Geometry check sheet. Reference: drawing and pictorial views, mm from the part's lowest x, y, z. A direction names the side the tool comes from. Round coordinates to 2 decimals unless told otherwise and drop trailing zeros. Write each loop counter-clockwise with the first axis right and the second up, starting at its lowest first coordinate (ties: lowest second). Pieces come first, ordered by that corner, then holes. Notation, with made-up numbers: (46, 83.5) -> (62, 83.5) arc R19 ccw to (62, 95.5) -> close; hole circle Ø1 at (62.5, 82.5). An arc over 180 degrees is marked (long way). Answer as a JSON object with one key per item and string values. Group by question number.
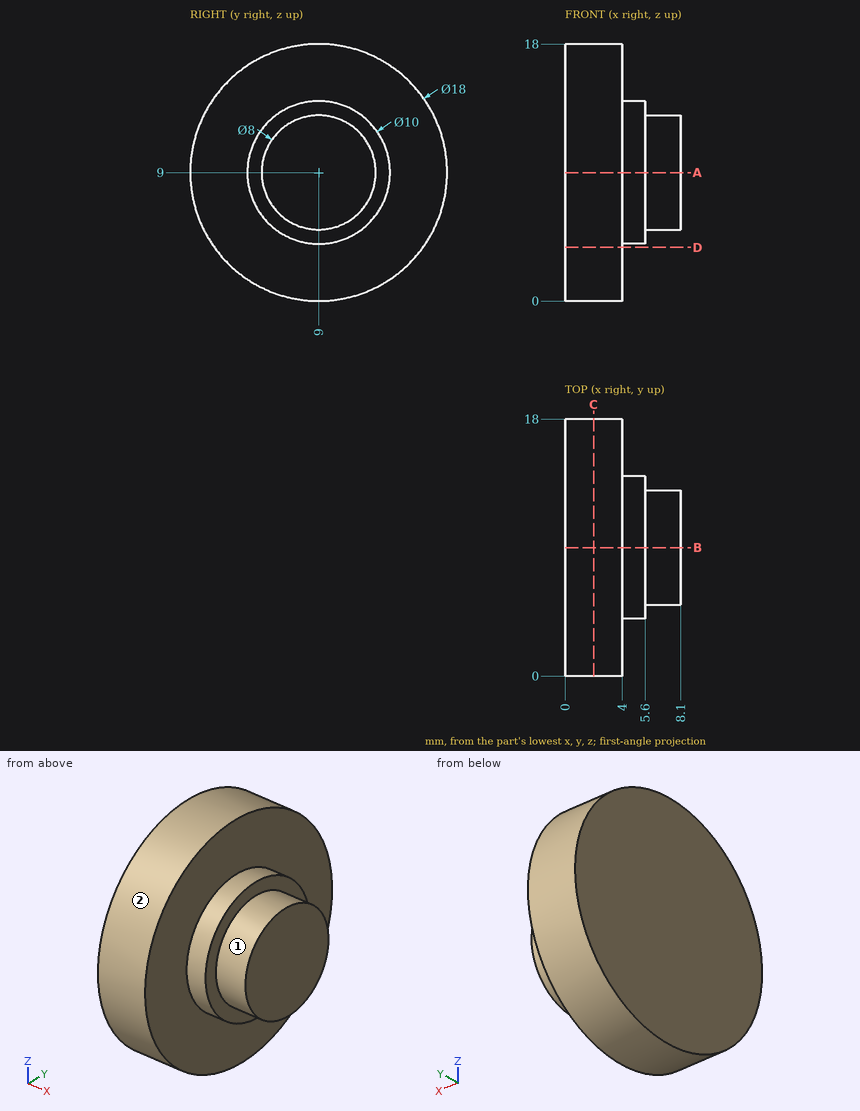
(1) Section check A-A on z = 9. Record the cut outline in (x, y).
(2) Access from +Z, -Z, +X, -X, +Y, -Y to the whole of each face (thin tool, end or side, straight path). Record for the marked faces 1 and 2.
(3) Go/stop test with flat-tipped pins: pin 1 Ø3 at (y, z) = (16, 4) entering from +X; pin 2 Ø3 at (x, y) = (6.5, 8) entering from -Z; pin 3 Ø4 at (x, y) = (4, 14.5) entering from -Z. Record where each tip stops, or that it passes through.
(4) Scan lines: line 1 along X through (y, z) = (11.25, 13.25); line 2 along X through (y, z) = (5.25, 12.5); line 3 along Z through (x, y) = (7, 12.25). Record each from-to range of solid material in increasing order.
(5) Section check D-D on z = 3.75. Record the cut outline in (x, y).
(6) Section check C-C on x = 2. Record the cut outline in (y, z).
Data:
{
 "1": {"outline": "(0, 0) -> (4, 0) -> (4, 4) -> (5.6, 4) -> (5.6, 5) -> (8.1, 5) -> (8.1, 13) -> (5.6, 13) -> (5.6, 14) -> (4, 14) -> (4, 18) -> (0, 18) -> close"},
 "2": {"face 1": "+X", "face 2": "+X, -X"},
 "3": {"pin 1": "stops at x = 4", "pin 2": "stops at z = 4", "pin 3": "stops at z = 0.71"},
 "4": {"line 1": "x = 0 to 5.6", "line 2": "x = 0 to 4", "line 3": "z = 6.67 to 11.33"},
 "5": {"outline": "(0, 1.69) -> (4, 1.69) -> (4, 16.31) -> (0, 16.31) -> close"},
 "6": {"outline": "circle Ø18 at (9, 9)"}
}
